```python
from build123d import *

# Parameters (mm, degrees)
SKETCH1_W           = 34.29
SKETCH1_H           = 12.7
SKETCH1_R           = 2.286
SKETCH1_R_2         = 1.778
BOSS_EXTRUDE1_DEPTH = 16.51
FILLET1_R           = 2.54
FILLET2_R           = 6.35
CUT_EXTRUDE2_DEPTH  = 5.08
CUT_EXTRUDE3_DEPTH  = 8.89


with BuildPart() as part:
    # Sketch1 → Boss-Extrude1 (new body)
    with BuildSketch(Plane(origin=(0, 0, 0), x_dir=(1, 0, 0), z_dir=(0, 1, 0))):
        with Locations((-1.905, 0)):
            Rectangle(SKETCH1_W, SKETCH1_H)
        with Locations(Location((-12.7, 1.27, 0), (0, 0, 270))):
            Circle(SKETCH1_R, mode=Mode.SUBTRACT)
        with Locations(Location((0, 0, 0), (0, 0, 270))):
            Circle(SKETCH1_R_2, mode=Mode.SUBTRACT)
        with Locations(Location((8.89, 0, 0), (0, 0, 270))):
            Circle(SKETCH1_R_2, mode=Mode.SUBTRACT)
    extrude(amount=BOSS_EXTRUDE1_DEPTH)

    # Fillet1
    fillet1_edges = [part.edges().sort_by_distance(p)[0] for p in [
        (-19.05, 8.255, -6.35),
        (15.24, 8.255, -6.35),
        (15.24, 8.255, 6.35),
    ]]
    fillet(fillet1_edges, radius=FILLET1_R)

    # Fillet2
    fillet2_edges = [part.edges().sort_by_distance(p)[0] for p in [
        (-19.05, 8.255, 6.35),
    ]]
    fillet(fillet2_edges, radius=FILLET2_R)

    # Sketch4 → Cut-Extrude2 (cut)
    with BuildSketch(Plane(origin=(0, 16.51, 0), x_dir=(1, 0, 0), z_dir=(0, 1, 0))):
        Polygon((-7.567356107, 1.27), (-10.133678053, 5.715), (-15.266321947, 5.715), (-17.832643893, 1.27), (-15.266321947, -3.175), (-10.133678053, -3.175), align=None)
    extrude(amount=-CUT_EXTRUDE2_DEPTH, mode=Mode.SUBTRACT)

    # Sketch5 → Cut-Extrude3 (cut)
    with BuildSketch(Plane(origin=(0, 11.43, 0), x_dir=(1, 0, 0), z_dir=(0, 1, 0))):
        Polygon((-9.356438934, 1.27), (-11.028219467, 4.165608823), (-14.371780533, 4.165608823), (-16.043561066, 1.27), (-14.371780533, -1.625608823), (-11.028219467, -1.625608823), align=None)
    extrude(amount=-CUT_EXTRUDE3_DEPTH, mode=Mode.SUBTRACT)


solid = part.part
```
The model under review builds one solid part; all positions refer to its coordinate system, in mm. A direction names the side the tool comes from. Give positions to 0.01 mm unless a question says otherwise; leave off trailing zeros. Write each loop counter-clockwise with the first axis right and the second up, starting at its lowest first coordinate (ties: lowest second). Pieces come first, ordered by that corner, then holes. Notation, with made-up numbers: (72, 9.5) - (116, 9.5) arc R34 cw to (116, 42.5) - close; hole circle Ø1 at (-0.5, -33.5). An arc over 180 degrees is marked (long way). Answer in a Markdown table with one row per item. Add a question column.
1. Wall thickness on line 1 along Z through (x, y) = (-12.7, 1.2); line 2 along X through (y, z) = (8.5, 1.5); line 3 along X through (y, z) = (0.6, -1.27): over which ranges is each line inside the solid? List them lowest first. Write a range as [from, to].
2. Tool access review of faces 1 (the flat face through (-10.204, 7.047, 0.198)), 2 (the cylindrical face through (-18.326, 8.371, -5.586)): name each direction out of +Z, -Z, +X, -X, +Y, -Y from which nothing blocks a thin tool from reaching the whole face with its end or side.
3. We need section D-D on z = -4.75. Write out the cut boundary in (x, y), then the cut area to 3 significant figures.
4. Draft analysis for pull direction Z (two halves, no side actions). For faces 3 (the flat face through (-15.196, 7.047, -2.738)), 4 (the flat face through (-2, 0, 0)), 5 (the flat face through (-2, 8, -6.35)), state which applies: +Z half, -Z half, draft (parallel to the pull), parting line (faces both ways), or undercut.
5. We need section A-A on y = 7.75. Write out the cut boundary in (x, z).
6. We need section B-B on x = 0. Write out the cut boundary in (y, z).
7. We need section C-C on y = 12.25. Write out the cut boundary in (x, z) (3 decimals), then the cut area to 3 significant figures.
8. Insertion check: P1, Ø6.5, axis at x = -11, z = -1.5, coming from the +Y side; P2, Ø1, axis at y = 4.5, z = -5, coming from the -X side. Each pin has a flat end and moves straight along its axis. Give the tip position at first contact, or say it passes through.
Ans:
| question | item | result |
|---|---|---|
| 1 | line 1 | z = [-6.35, -3.56], [1.02, 6.35] |
| 1 | line 2 | x = [-18.87, -14.44], [-10.96, -0.95], [0.95, 7.94], [9.84, 15.24] |
| 1 | line 3 | x = [-19.05, -14.99], [-10.41, -1.24], [1.24, 7.65], [10.13, 15.24] |
| 2 | face 1 | +Y |
| 2 | face 2 | -Z, -X, +Y, -Y |
| 3 | outline | (-18.87, 0) - (15.06, 0) - (15.06, 16.51) - (-9.58, 16.51) - (-9.58, 11.43) - (-15.82, 11.43) - (-15.82, 16.51) - (-18.87, 16.51) - close |
| 3 | area | 528 mm^2 |
| 4 | face 3 | undercut |
| 4 | face 4 | draft |
| 4 | face 5 | -Z half |
| 5 | outline | (-19.05, -3.81) arc R2.54 ccw to (-16.51, -6.35) - (12.7, -6.35) arc R2.54 ccw to (15.24, -3.81) - (15.24, 3.81) arc R2.54 ccw to (12.7, 6.35) - (-12.7, 6.35) arc R6.35 ccw to (-19.05, 0) - close; hole (-16.04, -1.27) - (-14.37, -4.17) - (-11.03, -4.17) - (-9.36, -1.27) - (-11.03, 1.63) - (-14.37, 1.63) - close; hole circle Ø3.56 at (0, 0); hole circle Ø3.56 at (8.89, 0) |
| 6 | outline | (0, -6.35) - (16.51, -6.35) - (16.51, -1.78) - (0, -1.78) - close; (0, 1.78) - (16.51, 1.78) - (16.51, 6.35) - (0, 6.35) - close |
| 7 | outline | (-19.05, -3.81) arc R2.54 ccw to (-16.51, -6.35) - (12.7, -6.35) arc R2.54 ccw to (15.24, -3.81) - (15.24, 3.81) arc R2.54 ccw to (12.7, 6.35) - (-12.7, 6.35) arc R6.35 ccw to (-19.05, 0) - close; hole (-17.833, -1.27) - (-15.266, -5.715) - (-10.134, -5.715) - (-7.567, -1.27) - (-10.134, 3.175) - (-15.266, 3.175) - close; hole circle Ø3.556 at (0, 0); hole circle Ø3.556 at (8.89, 0) |
| 7 | area | 334 mm^2 |
| 8 | P1 | stops at y = 16.51 |
| 8 | P2 | stops at x = -18.95 |
